Source: CAD feature listing. Evaluate the final solid. Frame: model axes, mm. A direction names the side the tool comes from. Coordinates: 2 decimals unless noted, no trailing zeros. Order: outer loops, then holes, each group sorted by start corner. A loop starts at its lowest first (then second) coordinate and runs counter-clockwise, first axis right, second up.
Item 1: Reachability of faces 1 (the flat face through (92, -1229, 15)), 2 (the flat face through (92, -1229, 0)), 3 (the cylindrical face through (93.458, -1265.514, 7.395)) from +Z, -Z, +X, -X, +Y, -Y: full face, straight path, thin tool, end or side. Return the list, or none.
Item 2: Section C-C on z = 8.5. Return the cut outline in (x, y).
Item 3: Contact query for flat-ended pins moving along their axis: P1, Ø3, axis at y = -1230.5, z = -59.5, coming from the +X side; P2, Ø12, axis at y = -1251.5, z = -26.5, coming from the +X side; P3, Ø8, axis at y = -1214, z = -110.5, coming from the -X side; P4, Ø5, axis at x = 69.5, z = -44.5, coming from the -Y side. Output: stop coordinate, or through.
Item 4: Section D-D on y = -1199.5. Return the cut outline in (x, z).
Item 5: Section B-B on y = -1227.5. Return the cut outline in (x, z).
Item 6: Ray query, line 1 (Z direction, x = 103.5, y = -1210.5); line 2 (X direction, y = -1231, z = -12); line 3 (Y direction, x = 75.5, z = 26.5). Return the intervals inside material, ascending.
Item 7: Section A-A on x = 84.5. Return the cut outline in (y, z).
from build123d import *

# Parameters (mm, degrees)
SKETCH1_R                = 40
BOSS_EXTRUDE1_DEPTH      = 15
BOSS_EXTRUDE2_DEPTH      = 69
BOSS_EXTRUDE2_DEPTH_BACK = 209
SKETCH2_R                = 15


with BuildPart() as part:
    # Sketch1 → Boss-Extrude1 (new body)
    with BuildSketch(Plane.XY):
        with Locations((75, -1230.027041119)):
            Circle(SKETCH1_R)
    extrude(amount=BOSS_EXTRUDE1_DEPTH)

    # Sketch2 → Boss-Extrude2 (add, two sides: drawn at the far end of the back side and taken through both)
    with BuildSketch(Plane.XY.offset(15).offset(-BOSS_EXTRUDE2_DEPTH_BACK)):
        with Locations((75, -1230.027041119)):
            Circle(SKETCH2_R)
    extrude(amount=BOSS_EXTRUDE2_DEPTH + BOSS_EXTRUDE2_DEPTH_BACK)


solid = part.part
Answer list:
1. face 1: +Z
1. face 2: -Z
1. face 3: +Z, -Z
2. outline: circle Ø80 at (75, -1230.03)
3. P1: stops at x = 90
3. P2: passes through
3. P3: stops at x = 66.04
3. P4: stops at y = -1244.72
4. outline: (49.15, 0) - (100.85, 0) - (100.85, 15) - (49.15, 15) - close
5. outline: (35.08, 0) - (60.21, 0) - (60.21, -194) - (89.79, -194) - (89.79, 0) - (114.92, 0) - (114.92, 15) - (89.79, 15) - (89.79, 84) - (60.21, 84) - (60.21, 15) - (35.08, 15) - close
6. line 1: z = 0 to 15
6. line 2: x = 60.03 to 89.97
6. line 3: y = -1245.02 to -1215.04
7. outline: (-1268.88, 0) - (-1241.64, 0) - (-1241.64, -194) - (-1218.42, -194) - (-1218.42, 0) - (-1191.17, 0) - (-1191.17, 15) - (-1218.42, 15) - (-1218.42, 84) - (-1241.64, 84) - (-1241.64, 15) - (-1268.88, 15) - close
